```python
from build123d import *

# Parameters (mm, degrees)
SKETCH_1_W               = 150
SKETCH_1_H               = 80
EXTRUDE_1_DEPTH          = 4
CUT_EXTRUDE_2_DEPTH      = 12
CUT_EXTRUDE_2_DEPTH_BACK = 27
SKETCH_2_R               = 6
SKETCH_2_R_2             = 2.6


with BuildPart() as part:
    # 草图1 → 凸台-拉伸1 (new body)
    with BuildSketch(Plane.XY):
        with Locations((11.84459115, -3.937887846)):
            Rectangle(SKETCH_1_W, SKETCH_1_H)
    extrude(amount=EXTRUDE_1_DEPTH)

    # 草图2 → 切除-拉伸2 (cut, two sides: drawn at the far end of the back side and taken through both)
    with BuildSketch(Plane.XY.offset(4).offset(-CUT_EXTRUDE_2_DEPTH_BACK)):
        with Locations((48.84459115, 16.062112154)):
            Circle(SKETCH_2_R)
        with Locations((-53.15540885, -33.937887846)):
            Circle(SKETCH_2_R_2)
        with Locations((76.84459115, -33.937887846)):
            Circle(SKETCH_2_R_2)
    extrude(amount=CUT_EXTRUDE_2_DEPTH + CUT_EXTRUDE_2_DEPTH_BACK, mode=Mode.SUBTRACT)


solid = part.part
```
For this review, take the finished solid that the model builds, in its own axes (mm). Coordinates: 2 decimals unless noted, no trailing zeros. Write each loop counter-clockwise with the first axis right and the second up, starting at its lowest first coordinate (ties: lowest second). Pieces come first, ordered by that corner, then holes. Notation, with made-up numbers: (-16, -1.75) - (-3, -1.75) arc R6 ccw to (-3, 8.25) - close; hole circle Ø11 at (-36.5, -15). An arc over 180 degrees is marked (long way). Answer in a Markdown table with one row per item. Add a question column.
Q1. Draft analysis for pull direction X (two halves, no side actions). For faces 1 (the flat face through (-63.155, -4, 2)), 2 (the flat face through (86.845, -4, 2)), 3 (the flat face through (11, -43.938, 2)), 4 (the cylindrical face through (79.325, -33.157, 1.972)), state which applies: +X half, -X half, draft (parallel to the pull), parting line (faces both ways), or undercut.
Q2. For P1, Ø4, axis at x = -53.16, y = -33.94, coming from the +Z side, flat-tipped, find the tip position at first contact; note if it passes through.
Q3. We need section A-A, the plane x = 51.5. State the section outline as (y, z) points.
Q4. We need section B-B, the plane y = 13. State the section outline as (x, z) points, and give its area (3 significant figures).
Q5. For probe 1 along X at (y, z) = (16.5, 2); probe 2 along Y at (x, z) = (52.5, 3.85); probe 3 along X at (y, z) = (12.5, 2.5), list the stretches that pass through material, from the lowest coordinate up.
Answer list:
| question | item | result |
|---|---|---|
| 1 | face 1 | -X half |
| 1 | face 2 | +X half |
| 1 | face 3 | draft |
| 1 | face 4 | undercut |
| 2 | P1 | passes through |
| 3 | outline | (-43.94, 0) - (10.68, 0) - (10.68, 4) - (-43.94, 4) - close; (21.44, 0) - (36.06, 0) - (36.06, 4) - (21.44, 4) - close |
| 4 | outline | (-63.16, 0) - (43.68, 0) - (43.68, 4) - (-63.16, 4) - close; (54, 0) - (86.84, 0) - (86.84, 4) - (54, 4) - close |
| 4 | area | 559 mm2 |
| 5 | probe 1 | x = -63.16 to 42.86, 54.83 to 86.84 |
| 5 | probe 2 | y = -43.94 to 11.3, 20.82 to 36.06 |
| 5 | probe 3 | x = -63.16 to 44.02, 53.67 to 86.84 |
